Design review of the part built by this model. Coordinates are the model's own, in mm. A direction names the side the tool comes from. Give positions to 0.01 mm unless a question says otherwise; leave off trailing zeros. Order: outer loops, then holes, each group sorted by start corner. A loop starts at its lowest first (then second) coordinate and runs counter-clockwise, first axis right, second up. Notation, with made-up numbers: (-30.5, -22.5) -> (13.5, -22.5) arc R30 cw to (13.5, 9.5) -> close; hole circle Ø9 at (47.5, 39). An arc over 180 degrees is marked (long way). One line per item, written item: value.
from build123d import *

# Parameters (mm, degrees)
SKETCH_1_R          = 5.03
EXTRUDE_1_DEPTH     = 4
CUT_EXTRUDE_1_DEPTH = 4
SKETCH_4_W          = 4
SKETCH_4_H          = 8
EXTRUDE_2_DEPTH     = 4


with BuildPart() as part:
    # 草图1 → 凸台-拉伸1 (new body)
    with BuildSketch(Plane.XY):
        with BuildLine():
            Line((-59.1, 38.97114317), (-59.1, 2.206540881))
            Line((-59.1, 2.206540881), (-59.1, -35.646026533))
            Line((-59.1, -35.646026533), (-47.142774211, -35.646026533))
            ThreePointArc((-47.142774211, -35.646026533), (-45.399104316, -35.087258865), (-44.304971996, -33.619103399))
            Line((-44.304971996, -33.619103399), (-22.5, 29.97114317))
            ThreePointArc((-22.5, 29.97114317), (-14.057833007, 42.090408542), (-28.351857593, 45.808961734))
            Line((-28.351857593, 45.808961734), (-56.281374572, 45.808961734))
            Line((-56.281374572, 45.808961734), (-59.1, 45.808961734))
            Line((-59.1, 45.808961734), (-59.1, 42.814449543))
            Line((-59.1, 42.814449543), (-59.1, 38.97114317))
        make_face()
        with BuildLine():
            ThreePointArc((-35.014022641, 37.07877749), (-34.09949662, 36.993301041), (-33.253696548, 36.635130268))
            ThreePointArc((-33.253696548, 36.635130268), (-32.007498532, 35.093487817), (-31.994845854, 33.111188432))
            Line((-31.994845854, 33.111188432), (-43.262197785, 0.251999821))
            ThreePointArc((-43.262197785, 0.251999821), (-46.59325113, -1.734096056), (-49.1, 1.225076687))
            Line((-49.1, 1.225076687), (-49.1, 15.527048957))
            Line((-49.1, 15.527048957), (-49.1, 29.38821049))
            ThreePointArc((-49.1, 29.38821049), (-48.888683815, 30.494213466), (-48.284504946, 31.444405555))
            Line((-48.284504946, 31.444405555), (-44.278244198, 35.700663421))
            ThreePointArc((-44.278244198, 35.700663421), (-43.366317827, 36.361183979), (-42.275113824, 36.638980548))
            Line((-42.275113824, 36.638980548), (-35.014022641, 37.07877749))
        make_face(mode=Mode.SUBTRACT)
        with Locations((-22.5, 38.97114317)):
            Circle(SKETCH_1_R, mode=Mode.SUBTRACT)
    extrude(amount=EXTRUDE_1_DEPTH)

    # 草图2 → 切除-拉伸1 (cut)
    with BuildSketch(Plane.XY.offset(4)):
        Polygon((-59.1, -14.837441681), (-55.1, -14.837441681), (-55.1, -13.487441681), (-52.5, -13.487441681), (-52.5, -14.837441681), (-50.5, -14.837441681), (-50.5, -17.837441681), (-52.5, -17.837441681), (-52.5, -19.187441681), (-55.1, -19.187441681), (-55.1, -17.837441681), (-59.1, -17.837441681), align=None)
        Polygon((-59.1, 37.162558319), (-55.1, 37.162558319), (-55.1, 38.512558319), (-52.5, 38.512558319), (-52.5, 37.162558319), (-50.5, 37.162558319), (-50.5, 34.162558319), (-52.5, 34.162558319), (-52.5, 32.812558319), (-55.1, 32.812558319), (-55.1, 34.162558319), (-59.1, 34.162558319), align=None)
    extrude(amount=-CUT_EXTRUDE_1_DEPTH, mode=Mode.SUBTRACT)

    # 草图4 → 凸台-拉伸2 (add)
    with BuildSketch(Plane.ZY.offset(59.1)):
        with Locations((2, 9.659412515)):
            Rectangle(SKETCH_4_W, SKETCH_4_H)
    extrude(amount=EXTRUDE_2_DEPTH)


solid = part.part
Item 1: Add section A-A on x = -45.5. Give the boundary of the cut face in (y, z), plus the area to 3 significant figures.
Returned:
outline: (-35.16, 0) -> (-1.71, 0) -> (-1.71, 4) -> (-35.16, 4) -> close; (34.4, 0) -> (45.81, 0) -> (45.81, 4) -> (34.4, 4) -> close
area: 179 mm²
Item 2: Clearance check with flat-ended pins moving along their axes: P1, Ø5, axis at x = -36, y = -13.5, coming from the -Z side; P2, Ø1.5, axis at y = 17.5, z = 2, coming from the +X side; P3, Ø0.7, axis at y = -18.5, z = 2.5, coming from the -X side; P4, Ø1.5, axis at y = 8, z = 1.5, coming from the +X side. State where each tip first meets the part, or that it passes through.
Returned:
P1: z = 0
P2: x = -26.52
P3: x = -59.1
P4: x = -29.78
Item 3: Add section B-B on z = 0.8. Count the separate pieces of the cut face and the enclosed holes in it, plus the area to 3 significant figures.
Returned:
separate pieces: 1
enclosed holes: 2
area: 1,840 mm²
Item 4: Machinability: for faces 1 (the flat face through (-59.1, 42, 2)), 2 (the flat face through (-50.5, -16, 2)), 3 (the cylindrical face through (-46.535, -1.743, 1.972)), which of the approach directions +Z, -Z, +X, -X, +Y, -Y give a long, thin tool a straight path to every point of the face, cutting with its end or side? Answer none if there is none.
Returned:
face 1: +Z, -Z, -X, +Y
face 2: +Z, -Z, -X
face 3: +Z, -Z
Item 5: Add section C-C on y = -28. Give the boundary of the cut face in (x, z), plus the area to 3 significant figures.
Returned:
outline: (-59.1, 0) -> (-42.38, 0) -> (-42.38, 4) -> (-59.1, 4) -> close
area: 66.9 mm²
Item 6: Draft analysis for pull direction X (two halves, no side actions). For faces 4 (the flat face through (-50.5, 36, 2)), 5 (the flat face through (-61, 13.659, 2)), 6 (the cylindrical face through (-48.894, 30.479, 1.972)), 7 (the flat face through (-54, -19.187, 2)), state which applies: pulls with the +X half, pulls with the -X half, needs draft (parallel to the pull), parting line crosses it, or undercut.
Returned:
face 4: pulls with the -X half
face 5: needs draft
face 6: undercut
face 7: undercut
Item 7: To check wall thickness, follow line 1 along Y through (x, z) = (-58, 2.6); line 2 along X through (y, z) = (33.5, 1.6); line 3 along X through (y, z) = (26, 2.7). State the ranges of each line that lie inside material, in increasing order. Write a range as from..to.
Returned:
line 1: -35.65..-17.84, -14.84..34.16, 37.16..45.81
line 2: -59.1..-55.1, -52.5..-46.35, -31.89..-15.35
line 3: -59.1..-49.1, -34.43..-23.86
